from build123d import *

# Parameters (mm, degrees)
F0_W        = 37.869092077
F0_H        = 99.9836400151
F0_W_2      = 29.556363821
F0_H_2      = 88.9000073075
F1_DEPTH    = 15
F2_R        = 2
F3_W        = 33.869092077
F3_H        = 95.9836400151
F4_DEPTH    = 3
F6_D        = 6
F7_T1_DEPTH = 56.7819705518
F7_T3_DEPTH = 118.8965184899


# Not quite as in the source:
# - a fillet or chamfer that OpenCascade refuses, or shapes differently, is made with other operations: its cross-section is extruded or revolved along the edge and cut away or added


with BuildPart() as f1:
    # F0 (on Top) → F1 (new body)
    with BuildSketch(Plane.XY):
        Rectangle(F0_W, F0_H)
        Rectangle(F0_W_2, F0_H_2, mode=Mode.SUBTRACT)
    extrude(amount=F1_DEPTH)

    # F2
    f2_edges = [f1.edges().sort_by_distance(p)[0] for p in [
        (0, 49.99182, 15),
        (-18.934546, 0, 15),
        (0, -49.99182, 15),
        (18.934546, 0, 15),
        (-18.934546, 49.99182, 7.5),
        (-18.934546, -49.99182, 7.5),
        (18.934546, 49.99182, 7.5),
        (18.934546, -49.99182, 7.5),
        (14.778182, 0, 15),
        (-14.778182, 0, 15),
        (0, -44.450004, 15),
        (0, 44.450004, 15),
        (0, -44.450004, 0),
        (0, -49.99182, 0),
        (-14.778182, 0, 0),
        (18.934546, 0, 0),
        (14.778182, 0, 0),
        (0, 44.450004, 0),
        (0, 49.99182, 0),
        (-18.934546, 0, 0),
    ]]
    fillet(f2_edges, radius=F2_R)

    # F3 (on face) → F4 (join)
    with BuildSketch(Plane.XY.offset(15)):
        Rectangle(F3_W, F3_H)
    extrude(amount=F4_DEPTH)

    # F6 (through all)
    with Locations(Plane.YZ.offset(18.9345460385)):
        with Locations((-39.3181852996, 7.8409090638), (37.0454601943, 7.6136365533)):
            Hole(F6_D / 2)

    # F7: fillet of radius 5 on 4 edges, made by hand

    # F7_s2 → F7_t1 (cut)
    with BuildSketch(Plane.YZ.offset(-28.3909852759)):
        with BuildLine():
            ThreePointArc((-43.4092443126, 18), (-46.1478571001, 17.1833001327), (-47.9918200076, 15))
            Line((-47.9918200076, 15), (-47.9918200076, 18))
            Line((-47.9918200076, 18), (-43.4092443126, 18))
        make_face()
        with BuildLine():
            ThreePointArc((47.9918200076, 15), (46.1478571001, 17.1833001327), (43.4092443126, 18))
            Line((43.4092443126, 18), (47.9918200076, 18))
            Line((47.9918200076, 18), (47.9918200076, 15))
        make_face()
    extrude(amount=F7_T1_DEPTH, mode=Mode.SUBTRACT)

    # F7_s4 → F7_t3 (cut)
    with BuildSketch(Plane.XZ.offset(-59.448259245)):
        with BuildLine():
            ThreePointArc((16.9345460385, 15), (15.0905831311, 17.1833001327), (12.3519703436, 18))
            Line((12.3519703436, 18), (16.9345460385, 18))
            Line((16.9345460385, 18), (16.9345460385, 15))
        make_face()
        with BuildLine():
            ThreePointArc((-16.9345460385, 15), (-15.0905831311, 17.1833001327), (-12.3519703436, 18))
            Line((-12.3519703436, 18), (-16.9345460385, 18))
            Line((-16.9345460385, 18), (-16.9345460385, 15))
        make_face()
    extrude(amount=F7_T3_DEPTH, mode=Mode.SUBTRACT)


solid = f1.part
Geometry check sheet. Reference: the model listing, model coordinates, mm. A direction names the side the tool comes from. Give positions to 0.01 mm unless a question says otherwise; leave off trailing zeros. Order: outer loops, then holes, each group sorted by start corner. A loop starts at its lowest first (then second) coordinate and runs counter-clockwise, first axis right, second up. Notation, with made-up numbers: (56, 32.25) - (68, 32.25) arc R34 ccw to (68, 65.25) - close; hole circle Ø10 at (51, 9). An arc over 180 degrees is marked (long way). Answer as a JSON object with one key per item and string values.
(1) Tool access check on faces 1 (the flat face through (18.935, -1, 7)), 2 (the cylindrical face through (-15.35, 0.65, 0.6)), 3 (the cylindrical face through (0.23, -45.02, 14.4)). Record the directions out of +Z, -Z, +X, -X, +Y, -Y that give a thin tool (end or side, any length) a straight path to the whole face; none if there is none.
Report:
{"face 1": "+Z, -Z, +X, +Y, -Y", "face 2": "-Z", "face 3": "none"}
(2) Cross-section at D-D (z = 16.25). Record the cut outline in (x, y).
Report:
{"outline": "(-16.15, -47.21) - (16.15, -47.21) - (16.15, 47.21) - (-16.15, 47.21) - close"}
(3) Cross-section at B-B (y = -39). Record the cut outline in (x, z), then the cut area to 3 significant figures.
Report:
{"outline": "(-18.93, 2) arc R2 ccw to (-16.93, 0) - (-16.78, 0) arc R2 ccw to (-14.78, 2) - (-14.78, 4.86) - (-18.93, 4.86) - close; (-18.93, 10.82) - (-14.78, 10.82) - (-14.78, 13) arc R2 ccw to (-16.78, 15) - (16.78, 15) arc R2 ccw to (14.78, 13) - (14.78, 10.82) - (18.93, 10.82) - (18.93, 13) arc R2 ccw to (16.93, 15) arc R5 ccw to (12.35, 18) - (-12.35, 18) arc R5 ccw to (-16.93, 15) arc R2 ccw to (-18.93, 13) - close; (14.78, 2) arc R2 ccw to (16.78, 0) - (16.93, 0) arc R2 ccw to (18.93, 2) - (18.93, 4.86) - (14.78, 4.86) - close", "area": "162 mm^2"}
(4) Draft check along X on faces 4 (the cylindrical face through (18.333, 49.421, 7.577)), 5 (the flat face through (-18.935, -1, 7)), 6 (the flat face through (0, 44.45, 7)), 7 (the cylindrical face through (16.83, -42.09, 6.69)). Enter one of: released by +X, released by -X, zero draft, split by the parting line, or undercut.
Report:
{"face 4": "released by +X", "face 5": "released by -X", "face 6": "undercut", "face 7": "zero draft"}
(5) Material ranges on line 1 (X direction, y = -11, z = 12); line 2 (Y direction, x = 3, z = 3.25); line 3 (Z direction, x = -5, y = 38.5), recorded low to high.
Report:
{"line 1": "-18.93 to -14.78, 14.78 to 18.93", "line 2": "-49.99 to -44.45, 44.45 to 49.99", "line 3": "15 to 18"}
(6) Cross-section at C-C (y = -19.5). Record the cut outline in (x, z).
Report:
{"outline": "(-18.93, 2) arc R2 ccw to (-16.93, 0) - (-16.78, 0) arc R2 ccw to (-14.78, 2) - (-14.78, 13) arc R2 ccw to (-16.78, 15) - (16.78, 15) arc R2 ccw to (14.78, 13) - (14.78, 2) arc R2 ccw to (16.78, 0) - (16.93, 0) arc R2 ccw to (18.93, 2) - (18.93, 13) arc R2 ccw to (16.93, 15) arc R5 ccw to (12.35, 18) - (-12.35, 18) arc R5 ccw to (-16.93, 15) arc R2 ccw to (-18.93, 13) - close"}
(7) Depth check by flat-ended pin: pin 1 Ø3.5 at (y, z) = (37.05, 7.61) entering from -X; pin 2 Ø9.5 at (y, z) = (37.05, 7.61) entering from +X. Enter the tip coordinate at first touch or a pass-through.
Report:
{"pin 1": "through", "pin 2": "x = 18.93"}
(8) Cross-section at A-A (x = -9.5). Record the cut outline in (y, z), then the cut area to 3 significant figures.
Report:
{"outline": "(-49.99, 2) arc R2 ccw to (-47.99, 0) - (-46.45, 0) arc R2 ccw to (-44.45, 2) - (-44.45, 13) arc R2 ccw to (-46.45, 15) - (46.45, 15) arc R2 ccw to (44.45, 13) - (44.45, 2) arc R2 ccw to (46.45, 0) - (47.99, 0) arc R2 ccw to (49.99, 2) - (49.99, 13) arc R2 ccw to (47.99, 15) arc R5 ccw to (43.41, 18) - (-43.41, 18) arc R5 ccw to (-47.99, 15) arc R2 ccw to (-49.99, 13) - close", "area": "440 mm^2"}
